CAD build for the part. Positions are in the model's coordinates, mm. Face numbers are marked on the shaded views. A direction names the side the tool comes from. Coordinates: 2 decimals unless noted, no trailing zeros. Loops run counter-clockwise (first coordinate to the right, second up) from the corner with the lowest first, then second, coordinate; pieces in that order, holes last. Notation, with made-up numbers: (67.5, 69) -> (111.5, 69) arc R7 cw to (111.5, 73) -> close; hole circle Ø11 at (-12, -35.5). An arc over 180 degrees is marked (long way). Write each question's results on one line, items separated by ' | '.
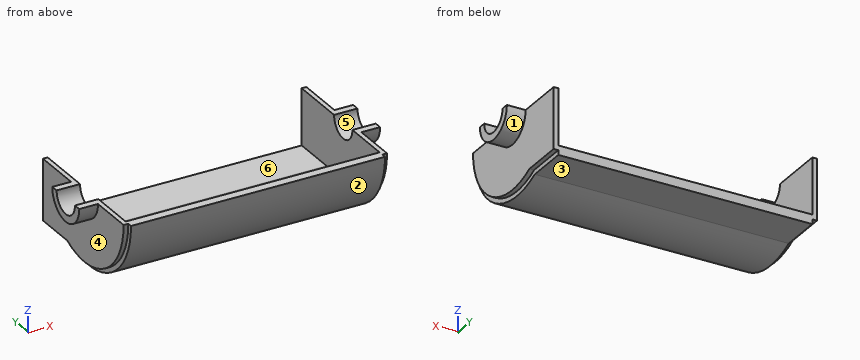
from build123d import *

# Parameters (mm, degrees)
Y_KSEKLIK_EKSTR_ZYON1_DEPTH = 20
Y_KSEKLIK_EKSTR_ZYON2_DEPTH = 5
EKSTR_ZYON_NCE4_DEPTH       = 271


with BuildPart() as part:
    # izim1 → Y_kseklik-Ekstr_zyon1 (new body)
    with BuildSketch(Plane(origin=(0, 0, 0), x_dir=(0, 0, -1), z_dir=(1, 0, 0))):
        with BuildLine():
            Line((0, 25), (0, 17))
            ThreePointArc((0, 17), (17, 0), (0, -17))
            Line((0, -17), (0, -25))
            ThreePointArc((0, -25), (25, 0), (0, 25))
        make_face()
    extrude(amount=Y_KSEKLIK_EKSTR_ZYON1_DEPTH)

    # izim2 → Y_kseklik-Ekstr_zyon2 (add)
    with BuildSketch(Plane(origin=(20, 0, 0), x_dir=(0, 0, -1), z_dir=(1, 0, 0))):
        with BuildLine():
            Line((0, 17), (0, 77))
            Line((0, 77), (65, 77))
            Line((65, 77), (65, 32.113081447))
            ThreePointArc((65, 32.113081447), (61.581037686, -38.262590053), (0, -72.5))
            Line((0, -72.5), (0, -17))
            ThreePointArc((0, -17), (17, 0), (0, 17))
        make_face()
    extrude(amount=Y_KSEKLIK_EKSTR_ZYON2_DEPTH)


with BuildPart() as body_2:
    # Aynalama4: mirrored copy
    add(part.part.mirror(Plane(origin=(160.5, 0, 0), x_dir=(0, 0, 1), z_dir=(1, 0, 0))))


with BuildPart() as part_1:
    add(part.part)

    add(body_2.part)  # Ekstr_zyon-_nce4 merges body 2
    # izim9 → Ekstr_zyon-_nce4 (add)
    with BuildSketch(Plane(origin=(25, 0, 0), x_dir=(0, 0, -1), z_dir=(1, 0, 0))):
        with BuildLine():
            ThreePointArc((0, -67.5), (57.634938288, -35.134938288), (60, 30.923292192))
            Line((60, 30.923292192), (60, 77))
            Line((60, 77), (70, 77))
            Line((70, 77), (70, 33.260336739))
            ThreePointArc((70, 33.260336739), (65.513075402, -41.4039485), (0, -77.5))
            Line((0, -77.5), (0, -67.5))
        make_face()
    extrude(amount=EKSTR_ZYON_NCE4_DEPTH)


solid = part_1.part
1) Two-plate mould, pull along X, no slides. Class the marked faces 4, 5 and 6: pulls with the +X half, pulls with the -X half, needs draft (parallel to the pull), parting line crosses it, or undercut.
Outcome:
face 4: pulls with the -X half | face 5: needs draft | face 6: undercut
2) Slice it at A-A (y = 0). Write the cut outline in (x, z), then the cut area to 4 significant figures.
Outcome:
outline: (0, -25) -> (20, -25) -> (20, -72.5) -> (25, -72.5) -> (25, -77.5) -> (296, -77.5) -> (296, -72.5) -> (301, -72.5) -> (301, -25) -> (321, -25) -> (321, -17) -> (296, -17) -> (296, -67.5) -> (25, -67.5) -> (25, -17) -> (0, -17) -> close | area: 3,585 mm^2
3) Slice it at C-C (z = -28). Write the cut outline in (x, y).
Outcome:
outline: (20, -66.87) -> (25, -66.87) -> (25, -72.27) -> (296, -72.27) -> (296, -66.87) -> (301, -66.87) -> (301, 77) -> (296, 77) -> (296, -61.42) -> (25, -61.42) -> (25, 77) -> (20, 77) -> close
4) Pin check, flat tips, straight feed: pin 1 (2.5 mm diameter, centred on x = 298.5, y = 54, fed in from -Z); pin 2 (6 mm diameter, centred on x = 196.5, y = -22, fed in from +Z); pin 3 (8 mm diameter, centred on y = 40, z = -13.5, fed in from -X). Stop position of each tip, or through.
Outcome:
pin 1: stops at z = -65 | pin 2: stops at z = -62.7 | pin 3: stops at x = 20
5) Drill centre lines: L1, parallel to X at y = 70, z = -27.5; L2, parallel to X at y = 6, z = -22; L3, parallel to X at y = -40, z = -58.5. Where is each one in solid material? Low to high. Write a range as from..to.
Outcome:
L1: x = 20..25, 296..301 | L2: x = 0..25, 296..321 | L3: x = 20..301
6) Slice it at B-B (z = -43). Write the cut outline in (x, y), then the cut area to 3 significant figures.
Outcome:
outline: (20, -58.37) -> (25, -58.37) -> (25, -64.48) -> (296, -64.48) -> (296, -58.37) -> (301, -58.37) -> (301, 77) -> (296, 77) -> (296, -52.03) -> (25, -52.03) -> (25, 77) -> (20, 77) -> close | area: 4,730 mm^2
7) Which spindle directions (+Z, -Z, +X, -X, +Y, -Y) get a long thin tool onto all of the face, cutting with end or side? Do the marked faces 1, 2 and 3. Say none if no direction does.
Outcome:
face 1: -Z, +X | face 2: -Z, +X, -X | face 3: -Z, +X, -X, +Y
